The model under review builds one solid part; all positions refer to its coordinate system, in mm. A direction names the side the tool comes from. Give positions to 0.01 mm unless a question says otherwise; leave off trailing zeros. Loops run counter-clockwise (first coordinate to the right, second up) from the corner with the lowest first, then second, coordinate; pieces in that order, holes last. Notation, with made-up numbers: M 8.5,31.5 L 62.5,31.5 A17 ccw 62.5,38.5 Z; hole C 68,64 d8. An arc over 180 degrees is marked long. One line per item, written item: value. Start each with the question number.
Q1. For pin 1 (16 mm diameter, centred on x = -190.5, z = 0, fed in from +Y); pin 2 (4 mm diameter, centred on x = -95, z = -32, fed in from +Y), all flat-tipped, find the tip position at first contact; note any pin that passes through.
Q2. We need section A-A on z = 0. Write out the cut boundary in (x, y).
Q3. We need section B-B on x = 190.5. Write out the cut boundary in (y, z).
Q4. We need section C-C on y = -2.5. Give the number of separate pieces and of enclosed holes in the cut face, plus the area to 3 significant figures.
Q5. For faces 1 (the face through (-97.2, -5.08, 31.8)), 2 (the face through (-195.45, -4.45, 0.22)), list the 3-axis set-ups (+Z, -Z, +X, -X, +Y, -Y) from which the entire face can be reached by the end or side of a thin tool; tool diameter is ignored.
```python
from build123d import *

# Parameters (mm, degrees)
F0_W     = 406.4
F0_H     = 75.692
F0_R     = 1.5875
F0_R_2   = 2.413
F0_R_3   = 4.953
F1_DEPTH = 9.017
F2_R     = 4.064
F3_DEPTH = 5.08


with BuildPart() as f1:
    # F0 (on Front) → F1 (new body)
    with BuildSketch(Plane.XZ):
        Rectangle(F0_W, F0_H)
        with Locations((-138.3665, -31.75)):
            Circle(F0_R, mode=Mode.SUBTRACT)
        with Locations((-126.3015, -31.75)):
            Circle(F0_R_2, mode=Mode.SUBTRACT)
        with Locations((-100.9015, -31.75)):
            Circle(F0_R, mode=Mode.SUBTRACT)
        with Locations((-94.5515, -31.75)):
            Circle(F0_R_2, mode=Mode.SUBTRACT)
        with Locations((94.5515, -31.75)):
            Circle(F0_R_2, mode=Mode.SUBTRACT)
        with Locations((100.9015, -31.75)):
            Circle(F0_R, mode=Mode.SUBTRACT)
        with Locations((126.3015, -31.75)):
            Circle(F0_R_2, mode=Mode.SUBTRACT)
        with Locations((138.3665, -31.75)):
            Circle(F0_R, mode=Mode.SUBTRACT)
        with Locations((-190.5, 0)):
            Circle(F0_R_3, mode=Mode.SUBTRACT)
        Circle(F0_R_3, mode=Mode.SUBTRACT)
        with Locations((-138.3665, 31.75)):
            Circle(F0_R, mode=Mode.SUBTRACT)
        with Locations((-126.3015, 31.75)):
            Circle(F0_R_2, mode=Mode.SUBTRACT)
        with Locations((-100.9015, 31.75)):
            Circle(F0_R, mode=Mode.SUBTRACT)
        with Locations((-94.5515, 31.75)):
            Circle(F0_R_2, mode=Mode.SUBTRACT)
        with Locations((190.5, 0)):
            Circle(F0_R_3, mode=Mode.SUBTRACT)
        with Locations((94.5515, 31.75)):
            Circle(F0_R_2, mode=Mode.SUBTRACT)
        with Locations((100.9015, 31.75)):
            Circle(F0_R, mode=Mode.SUBTRACT)
        with Locations((126.3015, 31.75)):
            Circle(F0_R_2, mode=Mode.SUBTRACT)
        with Locations((138.3665, 31.75)):
            Circle(F0_R, mode=Mode.SUBTRACT)
    extrude(amount=F1_DEPTH)

    # F2 (on face) → F3 (cut)
    with BuildSketch(Plane(origin=(0, 0, 0), x_dir=(-1, 0, 0), z_dir=(0, 1, 0))):
        with Locations((126.3015, 31.75)):
            Circle(F2_R)
        with Locations((94.5515, 31.75)):
            Circle(F2_R)
        with Locations((126.3015, -31.75)):
            Circle(F2_R)
        with Locations((94.5515, -31.75)):
            Circle(F2_R)
        with Locations((-126.3015, 31.75)):
            Circle(F2_R)
        with Locations((-94.5515, 31.75)):
            Circle(F2_R)
        with Locations((-94.5515, -31.75)):
            Circle(F2_R)
        with Locations((-126.3015, -31.75)):
            Circle(F2_R)
    extrude(amount=-F3_DEPTH, mode=Mode.SUBTRACT)


solid = f1.part
```
Solved:
1. pin 1: y = 0
1. pin 2: y = -5.08
2. outline: M -203.2,-9.02 L -195.45,-9.02 L -195.45,0 L -203.2,0 Z; M -185.55,-9.02 L -4.95,-9.02 L -4.95,0 L -185.55,0 Z; M 4.95,-9.02 L 185.55,-9.02 L 185.55,0 L 4.95,0 Z; M 195.45,-9.02 L 203.2,-9.02 L 203.2,0 L 195.45,0 Z
3. outline: M -9.02,-37.85 L 0,-37.85 L 0,-4.95 L -9.02,-4.95 Z; M -9.02,4.95 L 0,4.95 L 0,37.85 L -9.02,37.85 Z
4. separate pieces: 1
4. enclosed holes: 19
4. area: 30,100 mm2
5. face 1: +Y
5. face 2: +Y, -Y
